```python
from build123d import *

# Parameters (mm, degrees)
SKETCH_1_W          = 85
SKETCH_1_H          = 75
EXTRUDE_1_DEPTH     = 1.6
CUT_EXTRUDE_1_REACH = 58.701
SKETCH_2_R          = 1.65
CHAMFER_2_SIZE      = 3
CHAMFER_3_SIZE      = 20
CUT_EXTRUDE_4_REACH = 58.701


with BuildPart() as part:
    # 草图1 → 凸台-拉伸1 (new body)
    with BuildSketch(Plane(origin=(0, 0, 0), x_dir=(1, 0, 0), z_dir=(0, 1, 0))):
        Rectangle(SKETCH_1_W, SKETCH_1_H)
    extrude(amount=EXTRUDE_1_DEPTH)

    # 草图2 → 切除-拉伸1 (cut, up to next)
    with BuildSketch(Plane(origin=(0, 1.6, 0), x_dir=(1, 0, 0), z_dir=(0, 1, 0)), mode=Mode.PRIVATE) as cut_extrude_1_sk1:
        with Locations(Location((-28, 20, 0), (0, 0, 270))):
            Circle(SKETCH_2_R)
    cut_extrude_1_tool1 = extrude(cut_extrude_1_sk1.sketch, amount=-CUT_EXTRUDE_1_REACH, mode=Mode.PRIVATE) & part.part
    # 草图2 → 切除-拉伸1 (cut, up to next)
    with BuildSketch(Plane(origin=(0, 1.6, 0), x_dir=(1, 0, 0), z_dir=(0, 1, 0)), mode=Mode.PRIVATE) as cut_extrude_1_sk2:
        with Locations(Location((-28, -20, 0), (0, 0, 270))):
            Circle(SKETCH_2_R)
    cut_extrude_1_tool2 = extrude(cut_extrude_1_sk2.sketch, amount=-CUT_EXTRUDE_1_REACH, mode=Mode.PRIVATE) & part.part
    # 草图2 → 切除-拉伸1 (cut, up to next)
    with BuildSketch(Plane(origin=(0, 1.6, 0), x_dir=(1, 0, 0), z_dir=(0, 1, 0)), mode=Mode.PRIVATE) as cut_extrude_1_sk3:
        with Locations(Location((28, 20, 0), (0, 0, 270))):
            Circle(SKETCH_2_R)
    cut_extrude_1_tool3 = extrude(cut_extrude_1_sk3.sketch, amount=-CUT_EXTRUDE_1_REACH, mode=Mode.PRIVATE) & part.part
    # 草图2 → 切除-拉伸1 (cut, up to next)
    with BuildSketch(Plane(origin=(0, 1.6, 0), x_dir=(1, 0, 0), z_dir=(0, 1, 0)), mode=Mode.PRIVATE) as cut_extrude_1_sk4:
        with Locations(Location((28, -20, 0), (0, 0, 270))):
            Circle(SKETCH_2_R)
    cut_extrude_1_tool4 = extrude(cut_extrude_1_sk4.sketch, amount=-CUT_EXTRUDE_1_REACH, mode=Mode.PRIVATE) & part.part
    add(cut_extrude_1_tool1.solids().sort_by_distance((-28, 1.6, -20))[0], mode=Mode.SUBTRACT)
    add(cut_extrude_1_tool2.solids().sort_by_distance((-28, 1.6, 20))[0], mode=Mode.SUBTRACT)
    add(cut_extrude_1_tool3.solids().sort_by_distance((28, 1.6, -20))[0], mode=Mode.SUBTRACT)
    add(cut_extrude_1_tool4.solids().sort_by_distance((28, 1.6, 20))[0], mode=Mode.SUBTRACT)

    # 倒角2
    chamfer_2_edges = [part.edges().sort_by_distance(p)[0] for p in [
        (-42.5, 0.8, -37.5),
        (42.5, 0.8, -37.5),
    ]]
    chamfer(chamfer_2_edges, length=CHAMFER_2_SIZE)

    # 倒角3
    chamfer_3_edges = [part.edges().sort_by_distance(p)[0] for p in [
        (42.5, 0.8, 37.5),
        (-42.5, 0.8, 37.5),
    ]]
    chamfer(chamfer_3_edges, length=CHAMFER_3_SIZE)

    # 草图7 → 切除-拉伸4 (cut, up to next)
    with BuildSketch(Plane(origin=(0, 1.6, 0), x_dir=(1, 0, 0), z_dir=(0, 1, 0)), mode=Mode.PRIVATE) as cut_extrude_4_sk1:
        Polygon((-35, -25), (-35, -20), (-42.5, -12.5), (-42.5, -17.5), align=None)
    cut_extrude_4_tool1 = extrude(cut_extrude_4_sk1.sketch, amount=-CUT_EXTRUDE_4_REACH, mode=Mode.PRIVATE) & part.part
    cut_extrude_4 = cut_extrude_4_tool1.solids().sort_by_distance((-38.75, 1.6, 18.75))[0]
    add(cut_extrude_4, mode=Mode.SUBTRACT)

    # 镜向1: 切除-拉伸4 across plane
    add(cut_extrude_4.mirror(Plane(origin=(0, 0, 0), x_dir=(0, 0, 1), z_dir=(1, 0, 0))), mode=Mode.SUBTRACT)


solid = part.part
```
Geometry: final body of the model. Coordinates: model frame, mm. Round coordinates to 2 decimals unless told otherwise and drop trailing zeros. Order: outer loops, then holes, each group sorted by start corner. A loop starts at its lowest first (then second) coordinate and runs counter-clockwise, first axis right, second up. Notation, with made-up numbers: M 17.5,56.5 L 32.5,56.5 A15 ccw 32.5,66.5 Z; hole C -28.5,-31 d7. An arc over 180 degrees is marked long. Use one line per item in the form item = value. Start each with the question number.
Q1. Material intervals for line 1 (X direction, y = 1.15, z = -20); line 2 (X direction, y = 0.6, z = 20); line 3 (Z direction, x = 27, y = 0.95), sorted ascending. Write a range as [from, to].
Q2. Pin query (flat end, axial travel): pin 1 Ø2 at (x, z) = (28, -20) entering from -Y. Return the tip coordinate at first contact, or that it passes through.
Q3. Cut plane D-D (x = 31.5). Return loops of the section in (y, z).
Q4. Mould query, pull axis X, two halves, no side actions, for faces 1 (the face through (-39, 1, 16)), 2 (the face through (39, 1, 16)), 3 (the face through (-26.364, 0.811, 19.785)). Classes: +X half, -X half, draft (parallel to the pull), parting line (faces both ways), or undercut.
Q5. Cut plane A-A (z = -20). Return loops of the section in (x, y).
Q6. Cut plane C-C (y = 1.35). Return loops of the section in (x, z), and give its area (3 significant figures).
Q7. Cut plane B-B (x = -28). Return loops of the section in (y, z).
Geometry results:
q1.line_1 = [-42.5, -29.65], [-26.35, 26.35], [29.65, 42.5]
q1.line_2 = [-35, -29.65], [-26.35, 26.35], [29.65, 35]
q1.line_3 = [-37.5, -21.31], [-18.69, 18.69], [21.31, 33]
q2.pin_1 = through
q3.outline = M 0,-37.5 L 1.6,-37.5 L 1.6,28.5 L 0,28.5 Z
q4.face_1 = -X half
q4.face_2 = +X half
q4.face_3 = undercut
q5.outline = M -42.5,0 L -29.65,0 L -29.65,1.6 L -42.5,1.6 Z; M -26.35,0 L 26.35,0 L 26.35,1.6 L -26.35,1.6 Z; M 29.65,0 L 42.5,0 L 42.5,1.6 L 29.65,1.6 Z
q6.outline = M -42.5,-34.5 L -39.5,-37.5 L 39.5,-37.5 L 42.5,-34.5 L 42.5,12.5 L 35,20 L 35,25 L 22.5,37.5 L -22.5,37.5 L -35,25 L -35,20 L -42.5,12.5 Z; hole C -28,-20 d3.3; hole C -28,20 d3.3; hole C 28,-20 d3.3; hole C 28,20 d3.3
q6.area = 5,860 mm^2
q7.outline = M 0,-37.5 L 1.6,-37.5 L 1.6,-21.65 L 0,-21.65 Z; M 0,-18.35 L 1.6,-18.35 L 1.6,18.35 L 0,18.35 Z; M 0,21.65 L 1.6,21.65 L 1.6,32 L 0,32 Z
